Here's how the part is built. I have some questions about the finished solid (model axes, mm). Coordinates: 2 decimals unless noted, no trailing zeros. Write each loop counter-clockwise with the first axis right and the second up, starting at its lowest first coordinate (ties: lowest second). Pieces come first, ordered by that corner, then holes. Notation, with made-up numbers: (63.5, 43.25) -> (100.5, 43.25) arc R6 ccw to (100.5, 48.25) -> close; hole circle Ø1 at (-31, -35). An arc over 180 degrees is marked (long way). Use a Markdown table: item, result. Add a question column.
Item 1: Will these pins go through, and if not, where does the flat tip stop? pin 1 Ø9 at (x, y) = (36.25, 31.25) entering from +Z; pin 2 Ø5.5 at (x, z) = (-55.5, 2) entering from -Y; pin 3 Ø4 at (x, z) = (-57.5, 3.5) entering from +Y; pin 4 Ø12 at (y, z) = (5, -8.5) entering from -X.
Item 2: Imagine slicing it at B-B, the plane x = 33.5. Write out the boundary of the cut face in (y, z), and give its area (3 significant figures).
Item 3: Imagine slicing it at D-D, the plane y = -19.5. Write out the boundary of the cut face in (x, z).
Item 4: Imagine slicing it at A-A, the plane y = 31.25. Write out the boundary of the cut face in (x, z).
Item 5: If I drill on line 1 along Y through (x, z) = (36.25, 3.9); line 2 along Y through (x, z) = (0, 4.05); line 3 along Z through (x, y) = (50.5, 22), over which ranges is the centre line in solid material (lowest first)? Write a range as from..to.
Item 6: Imagine slicing it at C-C, the plane x = -51. Write out the boundary of the cut face in (y, z), and give its area (3 significant figures).
Autodesk Inventor part; units mm, degrees
ref_plane "YZ Plane" through (0, 0, 0) normal (1, 0, 0) x (0, 1, 0)
ref_plane "XZ Plane" through (0, 0, 0) normal (0, 1, 0) x (-1, 0, 0)
ref_plane "XY Plane" through (0, 0, 0) normal (0, 0, 1) x (1, 0, 0)
sketch "Sketch1" plane through (0, 0, 0) normal (0, 0, 1) x (1, 0, 0)
  line L0 (72.5, 62.5) -> (-72.5, 62.5)
  line L1 (-72.5, 62.5) -> (-72.5, -62.5)
  line L2 (-72.5, -62.5) -> (72.5, -62.5)
  line L3 (72.5, -62.5) -> (72.5, 62.5)
  line L4 (72.5, 62.5) -> (-72.5, -62.5) construction
  line L5 (-72.5, 62.5) -> (72.5, -62.5) construction
  point P0 (0, 0)
  dimension "d0" = 145
  dimension "d1" = 125
extrude "Extrusion1" add sketch "Sketch1" along normal blind 5
sketch "Sketch2" plane through (0, 0, 0) normal (0, 0, -1) x (-1, 0, 0)
  line L0 (-72.5, -62.5) -> (-72.5, 62.5)
  line L1 (-72.5, 62.5) -> (0, 0)
  line L2 (0, 0) -> (-72.5, -62.5)
  circle A0 centre (-36.25, 31.25) radius 5
  circle A1 centre (-36.25, -31.25) radius 5
  dimension "d4" = 10
  dimension "d5" = 10
extrude "Extrusion2" cut sketch "Sketch2" against normal blind 18.5 contours A1 L2 | L2 A1 | A0 L1 | L1 A0
sketch "Sketch3" plane through (0, 0, 0) normal (0, 0, -1) x (-1, 0, 0)
  line L0 (23.0298, -12.8396) -> (38.1112, -12.8396)
  line L1 (38.1112, -12.8396) -> (38.1112, 12.8396)
  line L2 (38.1112, 12.8396) -> (23.0298, 12.8396)
  line L3 (23.0298, 12.8396) -> (23.0298, -12.8396)
  line L4 (23.0298, -12.8396) -> (38.1112, 12.8396) construction
  line L5 (38.1112, -12.8396) -> (23.0298, 12.8396) construction
  point P0 (0, 0)
  point P1 (30.5705, 0)
extrude "Extrusion3" add sketch "Sketch3" along normal blind 15
shell "Shell1" thickness 2 removed faces 1 at (-23.0298, 4.2799, -5)
sketch "Sketch4" plane through (0, 0, 5) normal (0, 0, 1) x (1, 0, 0)
  line L0 (-72.5, -62.5) -> (72.5, -62.5)
  line L1 (0, 0) -> (-72.5, -62.5)
  line L2 (-36.25, -31.25) -> (0, -62.5)
  line L3 (-36.25, -31.25) -> (-36.25, -62.5)
  line L4 (-18.125, -46.875) -> (-18.125, -62.5)
  line L5 (0, 0) -> (72.5, -62.5)
  circle A0 centre (36.25, -31.25) radius 5
  line L6 (36.25, -31.25) -> (0, -62.5)
  line L7 (18.125, -46.875) -> (18.125, -62.5)
  line L8 (-18.125, -62.5) -> (18.125, -62.5)
  line L9 (18.125, -62.5) -> (18.125, -67.5)
  line L10 (18.125, -67.5) -> (-18.125, -67.5)
  line L11 (-18.125, -67.5) -> (-18.125, -62.5)
  dimension "d11" = 5
extrude "Extrusion4" add sketch "Sketch4" against normal blind 5 contours L0 L9 L10 L11
sketch "Sketch5" plane through (0, 0, 5) normal (0, 0, 1) x (1, 0, 0)
  line L0 (72.5, -62.5) -> (72.5, 62.5)
  line L1 (0, 0) -> (72.5, 62.5)
  line L2 (-72.5, 62.5) -> (-72.5, -62.5)
  line L3 (0, 0) -> (-72.5, 62.5)
  circle A0 centre (36.25, 31.25) radius 5
  line L4 (36.25, 31.25) -> (36.25, 62.5)
  line L5 (72.5, 62.5) -> (-72.5, 62.5)
  line L6 (-36.25, 31.25) -> (-36.25, 62.5)
  line L7 (-18.125, 15.625) -> (-18.125, 62.5)
  line L8 (36.25, 31.25) -> (0, 31.25)
  line L9 (18.125, 31.25) -> (18.125, 62.5)
  line L10 (18.125, 62.5) -> (-18.125, 62.5)
  line L11 (-18.125, 62.5) -> (-18.125, 67.5)
  line L12 (-18.125, 67.5) -> (18.125, 67.5)
  line L13 (18.125, 67.5) -> (18.125, 62.5)
  dimension "d14" = 5
extrude "Extrusion5" add sketch "Sketch5" against normal blind 5 contours L11 L12 L13 L5
sketch "Sketch6" plane through (0, 0, 5) normal (0, 0, 1) x (1, 0, 0)
  line L0 (-18.125, -62.5) -> (-18.125, -67.5)
  line L1 (18.125, -67.5) -> (18.125, -62.5)
  line L2 (-18.125, -62.5) -> (18.125, -62.5)
  circle A0 centre (0, -65) radius 1.5
  point P0 (0, 0)
  dimension "d17" = 3
extrude "Extrusion6" cut sketch "Sketch6" against normal blind 2.75
sketch "Sketch7" plane through (0, 0, 5) normal (0, 0, 1) x (1, 0, 0)
  line L0 (-18.125, 62.5) -> (-72.5, 62.5)
  line L1 (18.125, 62.5) -> (18.125, 67.5)
  line L2 (-18.125, 62.5) -> (18.125, 62.5)
  circle A0 centre (0, 65) radius 1.5
  point P0 (0, 0)
  dimension "d20" = 3
extrude "Extrusion7" cut sketch "Sketch7" against normal blind 2.75
properties part number "broomba base"
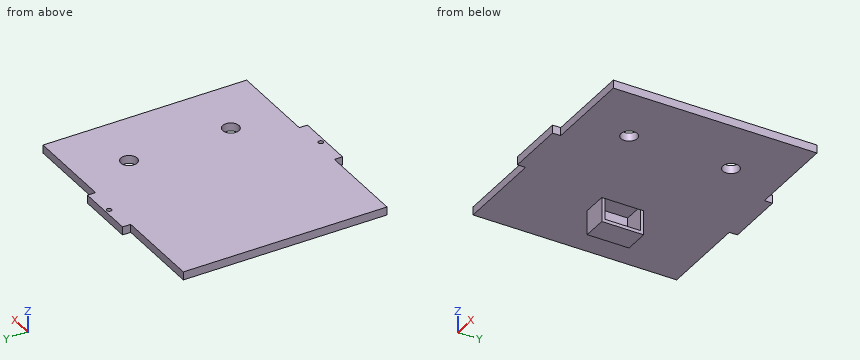
Ans:
| question | item | result |
|---|---|---|
| 1 | pin 1 | passes through |
| 1 | pin 2 | stops at y = -62.5 |
| 1 | pin 3 | stops at y = 62.5 |
| 1 | pin 4 | stops at x = -38.11 |
| 2 | outline | (-62.5, 0) -> (-35.43, 0) -> (-35.43, 5) -> (-62.5, 5) -> close; (-27.07, 0) -> (27.07, 0) -> (27.07, 5) -> (-27.07, 5) -> close; (35.43, 0) -> (62.5, 0) -> (62.5, 5) -> (35.43, 5) -> close; hole (-60.5, 2) -> (-37.69, 2) -> (-37.69, 3) -> (-60.5, 3) -> close; hole (-24.81, 2) -> (24.81, 2) -> (24.81, 3) -> (-24.81, 3) -> close; hole (37.69, 2) -> (60.5, 2) -> (60.5, 3) -> (37.69, 3) -> close |
| 2 | area | 446 mm^2 |
| 3 | outline | (-72.5, 0) -> (72.5, 0) -> (72.5, 5) -> (-72.5, 5) -> close; hole (-70.5, 2) -> (70.5, 2) -> (70.5, 3) -> (-70.5, 3) -> close |
| 4 | outline | (-72.5, 0) -> (31.25, 0) -> (31.25, 5) -> (-72.5, 5) -> close; (41.25, 0) -> (72.5, 0) -> (72.5, 5) -> (41.25, 5) -> close; hole (-70.5, 2) -> (29.25, 2) -> (29.25, 3) -> (-70.5, 3) -> close; hole (43.25, 2) -> (70.5, 2) -> (70.5, 3) -> (43.25, 3) -> close |
| 5 | line 1 | y = -62.5..-36.25, -26.25..26.25, 36.25..62.5 |
| 5 | line 2 | y = -67.5..-66.5, -63.5..63.5, 66.5..67.5 |
| 5 | line 3 | z = 0..2, 3..5 |
| 6 | outline | (-62.5, 0) -> (62.5, 0) -> (62.5, 5) -> (-62.5, 5) -> close; hole (-60.5, 2) -> (60.5, 2) -> (60.5, 3) -> (-60.5, 3) -> close |
| 6 | area | 504 mm^2 |
